```python
from build123d import *

# Parameters (mm, degrees)
SKETCH1_R                   = 51.94
BOSS_EXTRUDE1_DEPTH         = 50.8
CUT_EXTRUDE1_START          = -30
CUT_EXTRUDE1_DEPTH          = 31
SKETCH3_R                   = 5
CUT_EXTRUDE2_DEPTH          = 3
CIRPATTERN1_COUNT           = 3
CIRPATTERN1_COPY_1_SKETCH_R = 5
CIRPATTERN1_COPY_1_DEPTH    = 3
CIRPATTERN1_COPY_2_SKETCH_R = 5
CIRPATTERN1_COPY_2_DEPTH    = 3
FILLET2_R                   = 5
SKETCH6_R                   = 25.4
BOSS_EXTRUDE2_DEPTH         = 25.4


with BuildPart() as part:
    # Sketch1 → Boss-Extrude1 (new body)
    with BuildSketch(Plane(origin=(0, 0, 0), x_dir=(1, 0, 0), z_dir=(0, 1, 0))):
        Circle(SKETCH1_R)
    extrude(amount=BOSS_EXTRUDE1_DEPTH)

    # Sketch2 → Cut-Extrude1 (cut)
    with BuildSketch(Plane(origin=(0, 50.8, 0), x_dir=(1, 0, 0), z_dir=(0, 1, 0)).offset(CUT_EXTRUDE1_START)):
        with BuildLine():
            Line((302.928702249, 14.198513891), (49.96164332, 14.198513891))
            Line((49.96164332, 14.198513891), (32.527604999, 14.198513891))
            ThreePointArc((32.527604999, 14.198513891), (18.329091108, 0), (32.527604999, -14.198513891))
            Line((32.527604999, -14.198513891), (49.96164332, -14.198513891))
            Line((49.96164332, -14.198513891), (302.928702249, -14.198513891))
            Line((302.928702249, -14.198513891), (808.862820107, -14.198513891))
            Line((808.862820107, -14.198513891), (808.862820107, 14.198513891))
            Line((808.862820107, 14.198513891), (302.928702249, 14.198513891))
        make_face()
    cut_extrude1 = extrude(amount=CUT_EXTRUDE1_DEPTH, mode=Mode.SUBTRACT)

    # Sketch3 → Cut-Extrude2 (cut)
    with BuildSketch(Plane.XY.offset(-14.198513891)):
        with Locations((40.848803203, 39.398991639)):
            Circle(SKETCH3_R)
    cut_extrude2 = extrude(amount=-CUT_EXTRUDE2_DEPTH, mode=Mode.SUBTRACT)

    # Mirror1: Cut-Extrude2 across plane
    add(cut_extrude2.mirror(Plane.XY), mode=Mode.SUBTRACT)

    # CirPattern1: Cut-Extrude1, Cut-Extrude2 ×3 about axis
    cirpattern1_axis = Axis((0, 0, 0), (0, 1, 0))
    for i in range(1, CIRPATTERN1_COUNT):
        add(cut_extrude1.rotate(cirpattern1_axis, i * 360 / CIRPATTERN1_COUNT), mode=Mode.SUBTRACT)
        add(cut_extrude2.rotate(cirpattern1_axis, i * 360 / CIRPATTERN1_COUNT), mode=Mode.SUBTRACT)

    # CirPattern1 copy 1 sketch → CirPattern1 copy 1 (cut)
    with BuildSketch(Plane(origin=(12.296273726, 0, -7.099256946), x_dir=(-0.5, 0, -0.866025404), z_dir=(-0.866025404, 0, 0.5))):
        with Locations((40.848803203, -39.398991639)):
            Circle(CIRPATTERN1_COPY_1_SKETCH_R)
    extrude(amount=-CIRPATTERN1_COPY_1_DEPTH, mode=Mode.SUBTRACT)

    # CirPattern1 copy 2 sketch → CirPattern1 copy 2 (cut)
    with BuildSketch(Plane(origin=(-12.296273726, 0, -7.099256946), x_dir=(-0.5, 0, 0.866025404), z_dir=(0.866025404, 0, 0.5))):
        with Locations((40.848803203, -39.398991639)):
            Circle(CIRPATTERN1_COPY_2_SKETCH_R)
    extrude(amount=-CIRPATTERN1_COPY_2_DEPTH, mode=Mode.SUBTRACT)

    # Fillet2
    fillet2_edges = [part.edges().sort_by_distance(p)[0] for p in [
        (25.97, 50.8, 44.981359473),
        (-8.326038354, 50.8, 42.818149238),
        (-9.164545554, 50.8, 15.873458528),
        (-32.918585806, 50.8, 28.619635346),
        (-51.94, 50.8, 0),
        (-32.918585806, 50.8, -28.619635346),
        (-9.164545554, 50.8, -15.873458528),
        (-8.326038354, 50.8, -42.818149238),
        (25.97, 50.8, -44.981359473),
        (41.24462416, 50.8, 14.198513891),
        (18.329091108, 50.8, 0),
        (41.24462416, 50.8, -14.198513891),
    ]]
    fillet(fillet2_edges, radius=FILLET2_R)

    # Sketch6 → Boss-Extrude2 (add)
    with BuildSketch(Plane.XZ):
        Circle(SKETCH6_R)
    extrude(amount=BOSS_EXTRUDE2_DEPTH)


solid = part.part
```
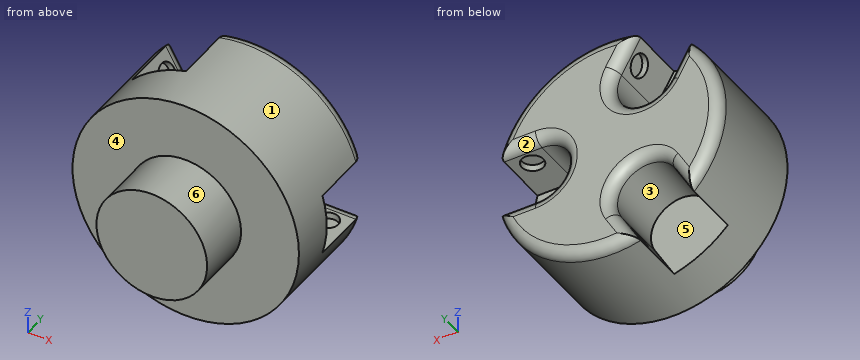
Read the model definition and answer for the solid it produces. Units are mm, in the model's axes. Face numbers are marked on the shaded views. A direction names the side the tool comes from. Give positions to 0.01 mm unless a question says otherwise; leave off trailing zeros. Order: outer loops, then holes, each group sorted by start corner. A loop starts at its lowest first (then second) coordinate and runs counter-clockwise, first axis right, second up. Notation, with made-up numbers: (75, 22.25) -> (106, 22.25) arc R3 cw to (106, 27.25) -> close; hole circle Ø11 at (23.25, 42). An arc over 180 degrees is marked (long way). One line per item, written item: value. Start each with the question number.
(1) The part is cut by section A-A (z = 0). Determine the outline of the cut face in (x, y).
(2) The part is cut by section C-C (y = -16). Determine the outline of the cut face in (x, z), and give its area (3 significant figures).
(3) Flat-ended cylindrical pins translate along their axes: P1, Ø4, axis at x = 24.5, y = 32.5, coming from the +Z side; P2, Ø5, axis at x = 40, y = 40.5, coming from the -Z side; P3, Ø2, axis at y = 16.5, z = -21, coming from the +X side (3 decimals). Find the tip coordinate at first contact, or state that the pin passes through.
(4) The part is cut by section D-D (y = 16.5). Determine the outline of the cut face in (x, z), and give its area (3 significant figures).
(5) For a pull along X with two mould halves and no side action, classify the marked faces 4, 5 and 6 as released by +X, released by -X, zero draft, split by the parting line, or undercut.
(6) The part is cut by section B-B (y = 32). Determine the outline of the cut face in (x, z).
(7) Straight lines are drawn through the part: L1, parallel to Z at x = -16, y = 23.5; L2, parallel to Y at x = -10, z = 31.5; L3, parallel to Y at x = -36.5, z = 25.5. For each, find the intervals that lie inside material, in ascending order.
(8) A tool of negligible diameter and unlimited length cuts with its end or side. For the marked faces 1, 2 and 3, from which of +Z, -Z, +X, -X, +Y, -Y can it reach the whole face along a straight path? Write none if from no direction.
Taken from the geometry:
1. outline: (-51.94, 0) -> (-25.4, 0) -> (-25.4, -25.4) -> (25.4, -25.4) -> (25.4, 0) -> (51.94, 0) -> (51.94, 20.8) -> (18.33, 20.8) -> (18.33, 45.8) arc R5 ccw to (13.33, 50.8) -> (-46.94, 50.8) arc R5 ccw to (-51.94, 45.8) -> close
2. outline: circle Ø50.8 at (0, 0)
2. area: 2,030 mm^2
3. P1: z = 46.81
3. P2: z = -35.94
3. P3: x = 47.935
4. outline: circle Ø103.88 at (0, 0)
4. area: 8,480 mm^2
5. face 4: zero draft
5. face 5: undercut
5. face 6: split by the parting line
6. outline: (-37.28, -36.17) -> (-28.56, -21.07) arc R14.2 cw to (-3.97, -35.27) -> (-12.68, -50.37) arc R51.94 ccw to (49.96, -14.2) -> (32.53, -14.2) arc R14.2 cw to (32.53, 14.2) -> (49.96, 14.2) arc R51.94 ccw to (-12.68, 50.37) -> (-3.97, 35.27) arc R14.2 cw to (-28.56, 21.07) -> (-37.28, 36.17) arc R51.94 ccw to start
7. L1: -13.97 to 13.97
7. L2: 0 to 20.8
7. L3: 0 to 50.79
8. face 1: +Y, -Y
8. face 2: +X, +Y
8. face 3: +Y
